Geometry check sheet. Reference: the model listing, model coordinates, mm. Give positions to 0.01 mm unless a question says otherwise; leave off trailing zeros. Write each loop counter-clockwise with the first axis right and the second up, starting at its lowest first coordinate (ties: lowest second). Pieces come first, ordered by that corner, then holes. Notation, with made-up numbers: (66, 70.5) - (90, 70.5) arc R18 cw to (90, 100.5) - close; hole circle Ø4 at (20.5, 44.25). An arc over 180 degrees is marked (long way). Write item = value, one per line. Start each with the question number.
(1) Draft check along Z on faces 1 (the cylindrical face through (7.715, 14.297, 0.301)), 2 (the flat face through (0, 30, 0)), 3 (the flat face through (4.5, 2, 1)). Enter one of: pulls with the +Z half, pulls with the -Z half, needs draft (parallel to the pull), parting line crosses it, or undercut.
(2) Section check C-C, the plane z = 1.5. Enter the section's corners in (x, y), plus the area to 3 significant figures.
(3) Section check B-B, the plane x = -2.25. Enter the section's corners in (y, z).
(4) Thickness scan on L1, parallel to X at y = 3, z = 1.15; L2, parallel to X at y = 21, z = 2.7; L3, parallel to Y at x = -1.5, z = 1.4. Record the ranges inside material, lowest first.
(5) Section check D-D, the plane y = 1.5. Enter the section's corners in (x, z), plus the area to 3 significant figures.
(6) Section check A-A, the plane y = 10.25. Enter the section's corners in (x, z), plus the area to 3 significant figures.
(7) Depth check by flat-ended pin: pin 1 Ø0.5 at (y, z) = (27.5, 2.5) entering from -X; pin 2 Ø0.8 at (x, z) = (2, 1.5) entering from -Y. Enter the tip coordinate at first touch or a pass-through.
```python
from build123d import *

# Parameters (mm, degrees)
BOSS_EXTRUDE1_DEPTH  = 3
SKETCH4_R            = 1.25
BOSS_EXTRUDE2_DEPTH  = 0.5
FILLET1_R            = 1
FILLET2_R            = 1
FILLET1_OF_MIRROR1_R = 1
FILLET2_OF_MIRROR1_R = 1


with BuildPart() as part:
    # Sketch3 → Boss-Extrude1 (new body)
    with BuildSketch(Plane.XY):
        Polygon((0, 30), (-8, 30), (-8, 18), (-8, 0), (-5, 0), (-5, 27), (0, 27), align=None)
    boss_extrude1 = extrude(amount=BOSS_EXTRUDE1_DEPTH)

    # Sketch4 → Boss-Extrude2 (add)
    with BuildSketch(Plane(origin=(-5, 0, 0), x_dir=(0, 0, -1), z_dir=(1, 0, 0))):
        with Locations(Location((-1.5, 1.5, 0), (0, 0, 270))):
            Circle(SKETCH4_R)
    boss_extrude2 = extrude(amount=BOSS_EXTRUDE2_DEPTH)

    # Fillet1
    fillet1_edges = [part.edges().sort_by_distance(p)[0] for p in [
        (-8, 15, 3),
        (-8, 15, 0),
    ]]
    fillet(fillet1_edges, radius=FILLET1_R)

    # Fillet2
    fillet2_edges = [part.edges().sort_by_distance(p)[0] for p in [
        (-8, 30, 1.5),
        (-2.5, 27, 3),
        (-7.707106781, 30, 2.707106781),
        (-7.707106781, 30, 0.292893219),
        (-2.5, 27, 0),
        (-3.5, 30, 3),
        (-3.5, 30, 0),
    ]]
    fillet(fillet2_edges, radius=FILLET2_R)

    # Mirror1: Boss-Extrude1, Boss-Extrude2 across plane
    add(boss_extrude1.mirror(Plane(origin=(0, 0, 0), x_dir=(0, 0, 1), z_dir=(1, 0, 0))))
    add(boss_extrude2.mirror(Plane(origin=(0, 0, 0), x_dir=(0, 0, 1), z_dir=(1, 0, 0))))

    # Fillet1 of Mirror1
    fillet1_of_mirror1_edges = [part.edges().sort_by_distance(p)[0] for p in [
        (8, 15, 3),
        (8, 15, 0),
    ]]
    fillet(fillet1_of_mirror1_edges, radius=FILLET1_OF_MIRROR1_R)

    # Fillet2 of Mirror1
    fillet2_of_mirror1_edges = [part.edges().sort_by_distance(p)[0] for p in [
        (8, 30, 1.5),
        (2.5, 27, 3),
        (7.707106781, 30, 2.707106781),
        (7.707106781, 30, 0.292893219),
        (2.5, 27, 0),
        (3.5, 30, 3),
        (3.5, 30, 0),
    ]]
    fillet(fillet2_of_mirror1_edges, radius=FILLET2_OF_MIRROR1_R)


solid = part.part
```
Model answer:
q1.face_1 = pulls with the -Z half
q1.face_2 = undercut
q1.face_3 = needs draft
q2.outline = (-8, 0) - (-5, 0) - (-5, 0.25) - (-4.5, 0.25) - (-4.5, 2.75) - (-5, 2.75) - (-5, 27) - (5, 27) - (5, 2.75) - (4.5, 2.75) - (4.5, 0.25) - (5, 0.25) - (5, 0) - (8, 0) - (8, 29) arc R1 ccw to (7, 30) - (-7, 30) arc R1 ccw to (-8, 29) - close
q2.area = 212 mm²
q3.outline = (27, 1) arc R1 ccw to (28, 0) - (29, 0) arc R1 ccw to (30, 1) - (30, 2) arc R1 ccw to (29, 3) - (28, 3) arc R1 ccw to (27, 2) - close
q4.L1 = -8 to -5, 5 to 8
q4.L2 = -7.71 to -5, 5 to 7.71
q4.L3 = 27 to 30
q5.outline = (-8, 1) arc R1 ccw to (-7, 0) - (-5, 0) - (-5, 0.25) - (-4.5, 0.25) - (-4.5, 2.75) - (-5, 2.75) - (-5, 3) - (-7, 3) arc R1 ccw to (-8, 2) - close; (4.5, 0.25) - (5, 0.25) - (5, 0) - (7, 0) arc R1 ccw to (8, 1) - (8, 2) arc R1 ccw to (7, 3) - (5, 3) - (5, 2.75) - (4.5, 2.75) - close
q5.area = 19.6 mm²
q6.outline = (-8, 1) arc R1 ccw to (-7, 0) - (-5, 0) - (-5, 3) - (-7, 3) arc R1 ccw to (-8, 2) - close; (5, 0) - (7, 0) arc R1 ccw to (8, 1) - (8, 2) arc R1 ccw to (7, 3) - (5, 3) - close
q6.area = 17.1 mm²
q7.pin_1 = -7.97
q7.pin_2 = 27
